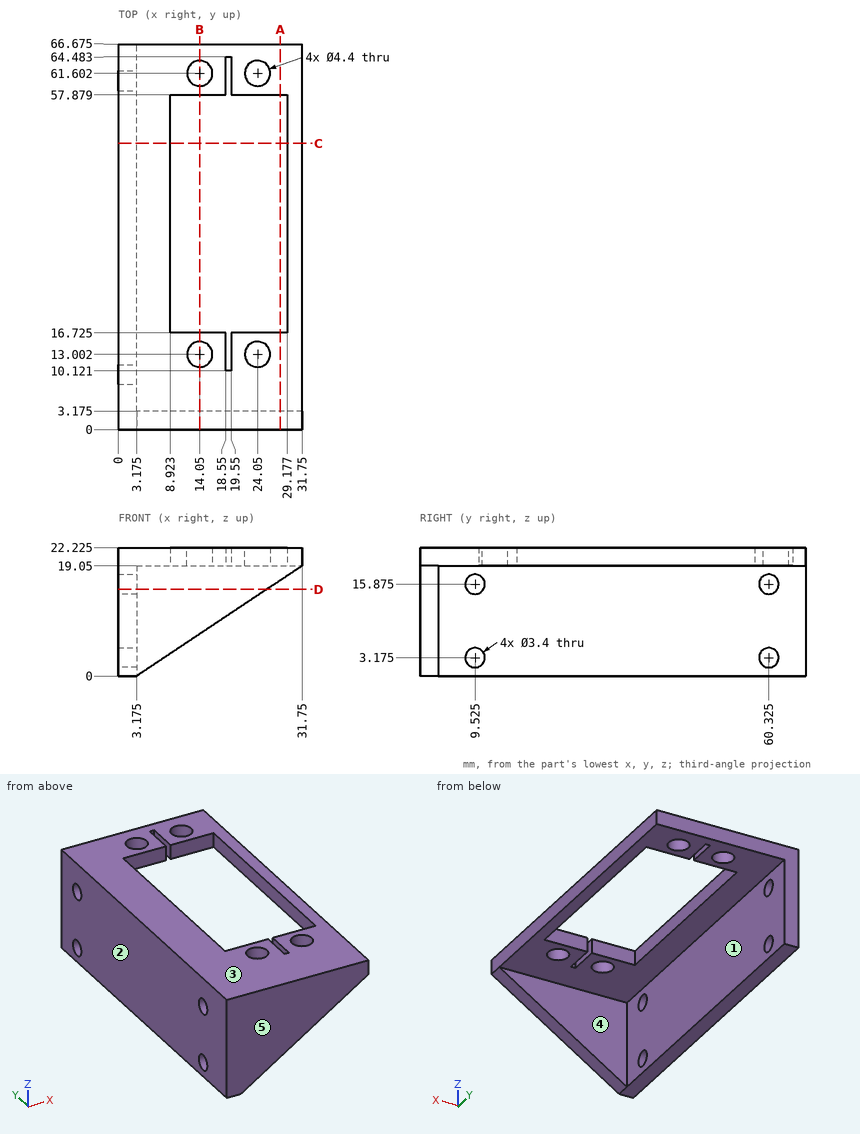
Can you work these out from the drawing? Everything is in mm from the part's minimum corner. A direction names the side the tool comes from. Round coordinates to 2 decimals unless told otherwise and drop trailing zeros. Order: outer loops, then holes, each group sorted by start corner. A loop starts at its lowest first (then second) coordinate and runs counter-clockwise, first axis right, second up. Notation, with made-up numbers: (65, 39.5) -> (80, 39.5) arc R10 ccw to (80, 55.5) -> close; hole circle Ø10 at (1.25, 82.5). An arc over 180 degrees is marked (long way). Return JSON: item names as keys, results as strings. Group by question number.
1. Will these pins go through, and if not, where does the flat tip stop? pin 1 (4 mm diameter, centred on y = 23.5, z = 14.5, fed in from +X) (3 decimals); pin 2 (5.5 mm diameter, centred on x = 23, z = 14, fed in from +Y) (3 decimals); pin 3 (2.5 mm diameter, centred on y = 60.325, z = 15.875, fed in from +X); pin 4 (12 mm diameter, centred on x = 23.5, y = 14, fed in from -Z).
2. We'd pull the mould along Y, two halves only. Please class the marked faces 3, 4 and 5: released by +Y, released by -Y, zero draft, split by the parting line, or undercut.
3. If we section it at B-B, the plane x = 14.05: Write out the boundary of the cut face in (y, z) (3 decimals).
4. If we section it at D-D, the plane z = 15: Write out the boundary of the cut face in (x, y) (3 decimals), then the cut area to 3 significant figures.
5. Which directions (+Z, -Z, +X, -X, +Y, -Y) give clear straight access to the entire face, cutting with the end or side of a thin tool? Please do the marked faces 1 and 2.
6. If we section it at A-A, the plane x = 28: Write out the boundary of the cut face in (y, z) (3 decimals).
7. If we section it at C-C, the plane y = 49.5: Write out the boundary of the cut face in (x, z) (3 decimals).
8. I need wall thicknesses on line 1 (Y direction, x = 24.05, z = 21.2) (3 decimals); line 2 (X direction, y = 29, z = 18.25) (3 decimals). Which ranges of each line are inside material? Lowest first, please. Write a range as [from, to].
Output values:
{
 "1": {"pin 1": "x = 3.175", "pin 2": "y = 3.175", "pin 3": "through", "pin 4": "z = 19.05"},
 "2": {"face 3": "zero draft", "face 4": "released by +Y", "face 5": "released by -Y"},
 "3": {"outline": "(0, 7.25) -> (3.175, 7.25) -> (3.175, 19.05) -> (10.802, 19.05) -> (10.802, 22.225) -> (0, 22.225) -> close; (15.202, 19.05) -> (16.725, 19.05) -> (16.725, 22.225) -> (15.202, 22.225) -> close; (57.879, 19.05) -> (59.402, 19.05) -> (59.402, 22.225) -> (57.879, 22.225) -> close; (63.802, 19.05) -> (66.675, 19.05) -> (66.675, 22.225) -> (63.802, 22.225) -> close"},
 "4": {"outline": "(0, 0) -> (25.675, 0) -> (25.675, 3.175) -> (3.175, 3.175) -> (3.175, 8.067) -> (0, 8.067) -> close; (0, 10.983) -> (3.175, 10.983) -> (3.175, 58.867) -> (0, 58.867) -> close; (0, 61.783) -> (3.175, 61.783) -> (3.175, 66.675) -> (0, 66.675) -> close", "area": "265 mm²"},
 "5": {"face 1": "-Z, +X, +Y", "face 2": "+Z, -Z, -X, +Y, -Y"},
 "6": {"outline": "(0, 16.55) -> (3.175, 16.55) -> (3.175, 19.05) -> (16.725, 19.05) -> (16.725, 22.225) -> (0, 22.225) -> close; (57.879, 19.05) -> (66.675, 19.05) -> (66.675, 22.225) -> (57.879, 22.225) -> close"},
 "7": {"outline": "(0, 0) -> (3.175, 0) -> (3.175, 19.05) -> (8.923, 19.05) -> (8.923, 22.225) -> (0, 22.225) -> close; (29.177, 19.05) -> (31.75, 19.05) -> (31.75, 22.225) -> (29.177, 22.225) -> close"},
 "8": {"line 1": "[0, 10.802], [15.202, 16.725], [57.879, 59.402], [63.802, 66.675]", "line 2": "[0, 3.175]"}
}
